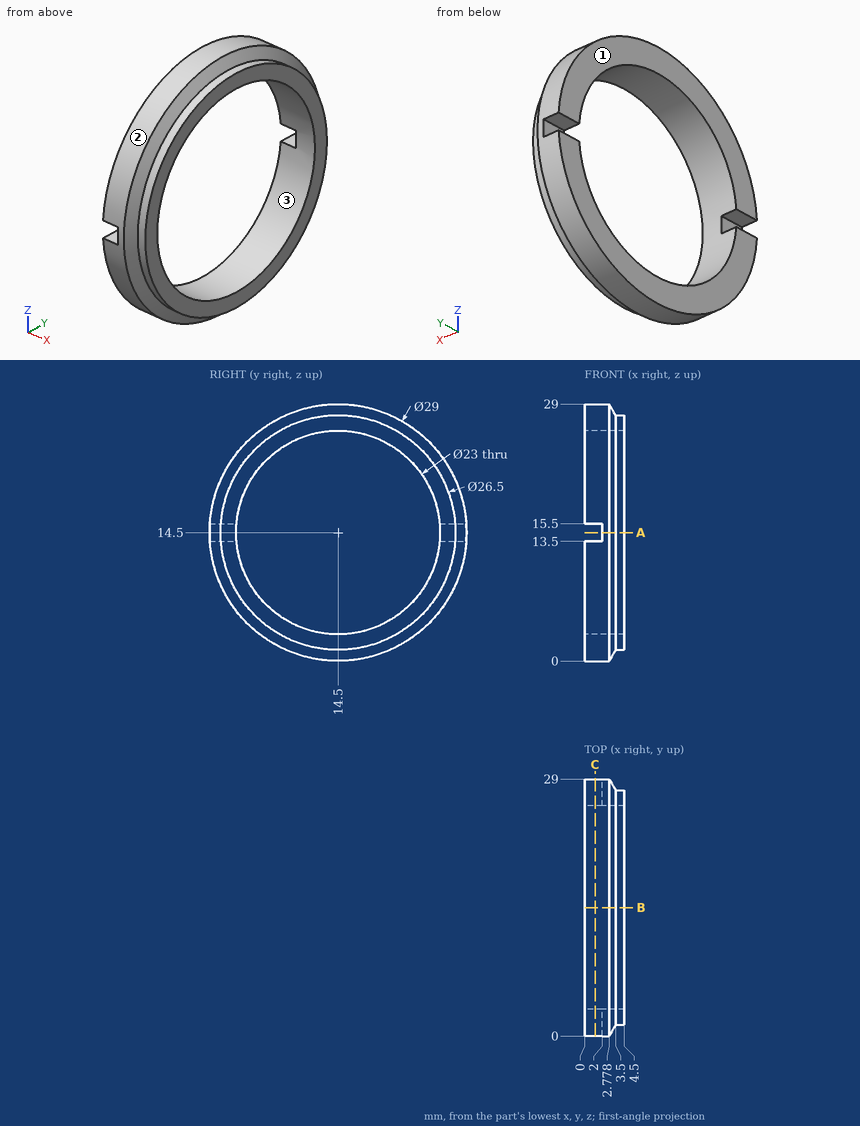
Geometry check sheet. Reference: drawing and pictorial views, mm from the part's lowest x, y, z. Coordinates: 2 decimals unless noted, no trailing zeros. Write each loop counter-clockwise with the first axis right and the second up, starting at its lowest first coordinate (ties: lowest second). Pieces come first, ordered by that corner, then holes. Notation, with made-up numbers: M 89,-34 L 136,-34 A21 cw 136,-1 Z; hole C 77,35 d5. An arc over 180 degrees is marked long. Use one line per item in the form item = value.
Item 1: Sectioned sample at A-A, the plane z = 14.5. Record the cut outline in (x, y), and give its area (3 significant figures).
Answer below:
outline = M 2,0 L 2.78,0 L 3.5,1.25 L 4.5,1.25 L 4.5,3 L 2,3 Z; M 2,26 L 4.5,26 L 4.5,27.75 L 3.5,27.75 L 2.78,29 L 2,29 Z
area = 11.6 mm^2
Item 2: Sectioned sample at C-C, the plane x = 1.2. Record the cut outline in (y, z) (1 decimal), and give its area (3 significant figures).
Answer below:
outline = M 0,13.5 A14.5 ccw 29,13.5 L 26,13.5 A11.5 cw 3,13.5 Z; M 0,15.5 L 3,15.5 A11.5 cw 26,15.5 L 29,15.5 A14.5 ccw Z
area = 233 mm^2
Item 3: Release check for a two-part mould opening along Y. For the marked faces 1, 2 and 3 record: pulls with the +Y half, pulls with the -Y half, needs draft (parallel to the pull), parting line crosses it, or undercut.
Answer below:
face_1 = needs draft
face_2 = parting line crosses it
face_3 = undercut
Item 4: Gauge pin test, flat ends, axial feed: pin 1 Ø2 at (x, y) = (0.5, 1.5) entering from +Z; pin 2 Ø0.6 at (x, y) = (1, 28) entering from +Z; pin 3 Ø6 at (y, z) = (25, 23.5) entering from -X; pin 4 Ø1 at (x, y) = (1, 1) entering from -Z. Record the tip position at first contact, or that the pin passes through.
Answer below:
pin_1 = 22.64
pin_2 = 20.5
pin_3 = 0
pin_4 = 8.08
Item 5: Material ranges on L1, parallel to Z at x = 1.45, y = 14.5; L2, parallel to Z at x = 1.2, y = 6.5 (1 decimal), recorded low to high. Write a range as from..to.
Answer below:
L1 = 0..3, 26..29
L2 = 2.4..6.2, 22.8..26.6
Item 6: Sectioned sample at B-B, the plane y = 14.5. Record the cut outline in (x, z).
Answer below:
outline = M 0,0 L 2.78,0 L 3.5,1.25 L 4.5,1.25 L 4.5,3 L 0,3 Z; M 0,26 L 4.5,26 L 4.5,27.75 L 3.5,27.75 L 2.78,29 L 0,29 Z
